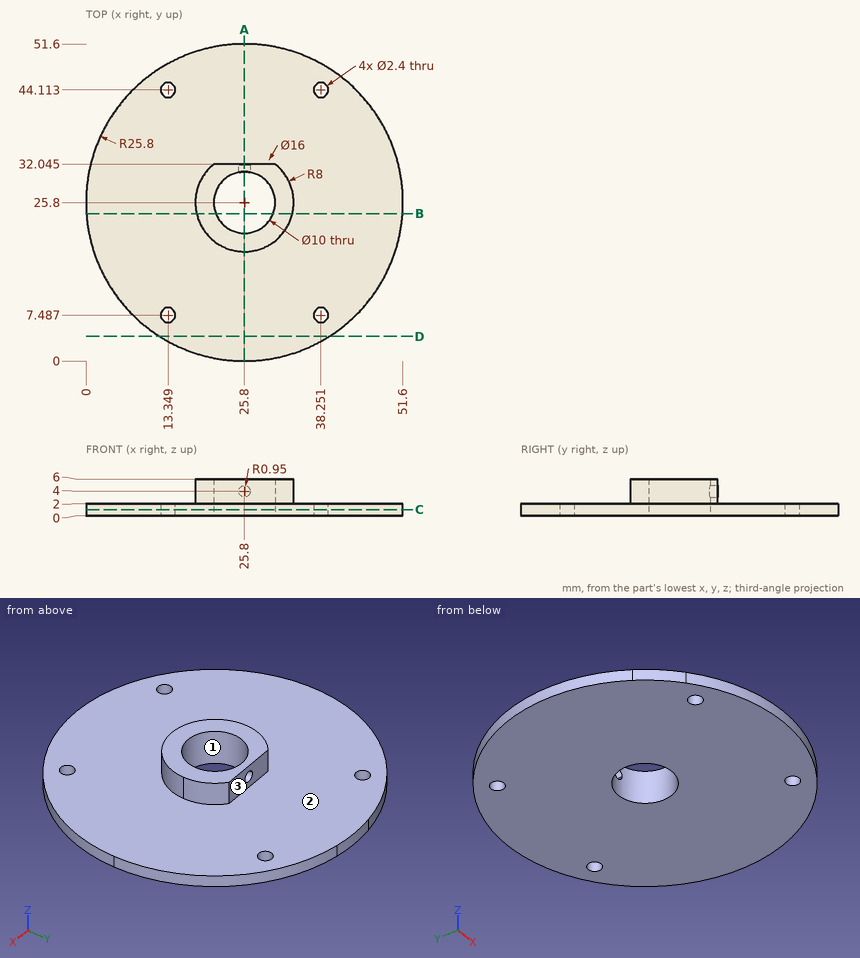
Verification items for this drawing (mm, ordinates from the low corner). Give positions to 0.01 mm unless a question says otherwise; leave off trailing zeros. Loops run counter-clockwise (first coordinate to the right, second up) from the corner with the lowest first, then second, coordinate; pieces in that order, holes last. Notation, with made-up numbers: M 3,44 L 17,44 A13 cw 17,61 Z; hole C 34.5,5.5 d4. An arc over 180 degrees is marked long. Answer as a JSON object with one key per item and string values. Group by question number.
Q1. Go/stop test with flat-tipped pins: P1, Ø1, axis at y = 21.5, z = 4, coming from the +X side; P2, Ø1.2, axis at x = 27.5, z = 4.5, coming from the +Y side (3 decimals); P3, Ø4, axis at x = 38.25, y = 44.11, coming from the +Z side; P4, Ø3, axis at y = 6.5, z = 4, coming from the -X side. Record where each tip stops, or that it passes through.
Q2. Release check for a two-part mould opening along Y. For the marked faces 1, 2 and 3 record: released by +Y, released by -Y, zero draft, split by the parting line, or undercut.
Q3. Material ranges on line 1 along Z through (x, y) = (3.5, 24.5); line 2 along Y through (x, z) = (25.5, 4) (1 decimal); line 3 along Y through (x, z) = (29, 1.5), recorded low to high. Write a range as [from, to].
Q4. Cross-section at D-D on y = 4. Record the cut outline in (x, z).
Q5. Cross-section at B-B on y = 24. Record the cut outline in (x, z) (1 decimal), then the cut area to 3 significant figures.
Q6. Cross-section at A-A on x = 25.8. Give the number of separate pieces and of enclosed holes in the cut face.
Q7. Cross-section at C-C on z = 1. Record the cut outline in (x, y), then the cut area to 3 significant figures.
Evaluation:
{
 "1": {"P1": "stops at x = 32.84", "P2": "stops at y = 32.045", "P3": "stops at z = 2", "P4": "passes through"},
 "2": {"face 1": "undercut", "face 2": "zero draft", "face 3": "released by +Y"},
 "3": {"line 1": "z = [0, 2]", "line 2": "y = [17.8, 20.8]", "line 3": "y = [0.2, 21.96], [29.64, 51.4]"},
 "4": {"outline": "M 12,0 L 39.6,0 L 39.6,2 L 12,2 Z"},
 "5": {"outline": "M 0.1,0 L 21.1,0 L 21.1,6 L 18,6 L 18,2 L 0.1,2 Z; M 30.5,0 L 51.5,0 L 51.5,2 L 33.6,2 L 33.6,6 L 30.5,6 Z", "area": "109 mm2"},
 "6": {"separate pieces": "3", "enclosed holes": "0"},
 "7": {"outline": "C 25.8,25.8 d51.6; hole C 13.35,7.49 d2.4; hole C 13.35,44.11 d2.4; hole C 25.8,25.8 d10; hole C 38.25,7.49 d2.4; hole C 38.25,44.11 d2.4", "area": "1,990 mm2"}
}
